For this review, take the finished solid that the model builds, in its own axes (mm). Face numbers are marked on the shaded views. A direction names the side the tool comes from. Coordinates: 2 decimals unless noted, no trailing zeros. Loops run counter-clockwise (first coordinate to the right, second up) from the corner with the lowest first, then second, coordinate; pieces in that order, holes last. Notation, with made-up numbers: (77, -28) -> (93, -28) arc R21 cw to (93, 6) -> close; hole circle Ø4 at (27.5, 65). An arc over 180 degrees is marked (long way). Answer in a Markdown table with one row per item.
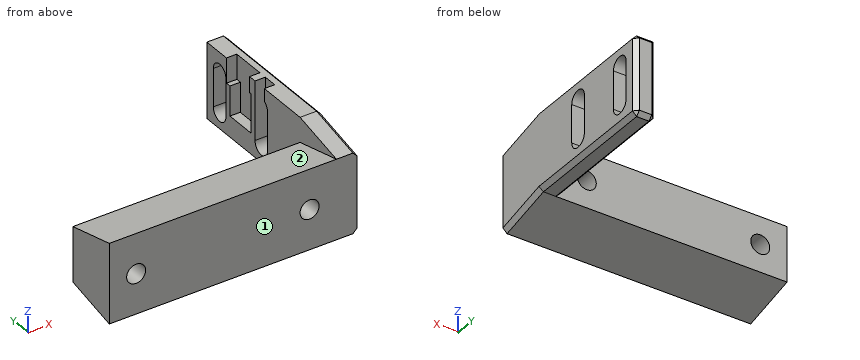
from build123d import *

# Parameters (mm, degrees)
PAD_DEPTH            = 55
SKETCH001_R          = 2.3
POCKET_DEPTH         = 13.001
PAD013_DEPTH         = 5
SKETCH023_W          = 7.25
SKETCH023_H          = 3.35
POCKET009_DEPTH      = 2.5
CHAMFER005_SIZE      = 1
BODY_PITCH_ANGLE     = 90
BODY_PLACEMENT_ANGLE = 90


with BuildPart() as part:
    # Sketch → Pad (new body)
    with BuildSketch(Plane.XZ):
        Polygon((0, 0), (19.3, 0), (16.3, 13), (3, 13), align=None)
    extrude(amount=PAD_DEPTH)

    # Sketch001 (on Face3 of Pad) → Pocket (cut, through all)
    with BuildSketch(Plane(origin=(0, 0, 13), x_dir=(-1, 0, 0), z_dir=(0, 0, 1))):
        with Locations((-9.65, 6.5)):
            Circle(SKETCH001_R)
        with Locations((-9.65, 48.5)):
            Circle(SKETCH001_R)
    extrude(amount=-POCKET_DEPTH, mode=Mode.SUBTRACT)

    # Sketch022 (on Face4 of Pocket) → Pad013 (join)
    with BuildSketch(Plane.XZ.offset(55)):
        Polygon((16.3, 13), (19.3, 0), (0, 0), (-3, 13), (-3, 47.3), (16.3, 47.3), (16.3, 44.3), (16.3, 24.3), (16.3, 18.3), align=None)
        with BuildLine():
            ThreePointArc((2.05, 44), (-0.2, 41.75), (2.05, 39.5))
            Line((2.05, 39.5), (11.25, 39.5))
            ThreePointArc((11.25, 39.5), (13.5, 41.75), (11.25, 44))
            Line((2.05, 44), (11.25, 44))
        make_face(mode=Mode.SUBTRACT)
        with BuildLine():
            ThreePointArc((2.05, 29.1), (-0.2, 26.85), (2.05, 24.6))
            Line((2.05, 24.6), (11.25, 24.6))
            ThreePointArc((11.25, 24.6), (13.5, 26.85), (11.25, 29.1))
            Line((2.05, 29.1), (11.25, 29.1))
        make_face(mode=Mode.SUBTRACT)
    extrude(amount=PAD013_DEPTH)

    # Sketch023 (on Face6 of Pad013) → Pocket009 (cut)
    with BuildSketch(Plane(origin=(0, -55, 0), x_dir=(1, 0, 0), z_dir=(0, 1, 0))):
        Polygon((10.25, -30.55), (10.25, -38.05), (3.05, -38.05), (3.05, -39.3), (-3, -39.3), (-3, -31.05), (0.85, -31.05), (0.85, -30.55), align=None)
        with Locations((0.625, -27.425)):
            Rectangle(SKETCH023_W, SKETCH023_H)
    extrude(amount=-POCKET009_DEPTH, mode=Mode.SUBTRACT)

    # Chamfer005
    chamfer005_edges = [part.edges().sort_by_distance(p)[0] for p in [
        (16.3, -57.5, 47.3),
        (6.65, -60, 47.3),
        (6.65, -55, 47.3),
        (-3, -57.5, 47.3),
        (-3, -60, 30.15),
        (16.3, -60, 30.15),
        (-1.5, -60, 6.5),
        (17.8, -60, 6.5),
        (16.3, -55, 30.15),
    ]]
    chamfer(chamfer005_edges, length=CHAMFER005_SIZE)


with BuildPart() as part_1:
    # Body pitch: moved
    add(part.part.rotate(Axis((0, 0, 0), (0, 1, 0)), BODY_PITCH_ANGLE))


with BuildPart() as part_2:
    # Body placement: moved
    add(part_1.part.moved(Location((-26, -25, -23))).rotate(Axis((-26, -25, -23), (0, 0, 1)), BODY_PLACEMENT_ANGLE))


solid = part_2.part
Item 1: For the marked faces 1 and 2, list the 3-axis set-ups (+Z, -Z, +X, -X, +Y, -Y) from which the entire face can be reached by the end or side of a thin tool; tool diameter is ignored.
Worked answers:
| item | result |
|---|---|
| face 1 | +Z, -Z, +X, -X, -Y |
| face 2 | +Z, -X, +Y |
Item 2: Take a section at B-B, the plane z = -32.5. State the section outline as (x, y) points, and give its area (3 significant figures).
Worked answers:
| item | result |
|---|---|
| outline | (-26, -25) -> (-21.8, -25) -> (-21.8, -12) -> (-26, -12) -> close; (-17.2, -25) -> (20.2, -25) -> (20.2, -12) -> (-17.2, -12) -> close; (24.8, -25) -> (34, -25) -> (34, -0.4) -> (29, -0.4) -> (29, -12) -> (24.8, -12) -> close; (29, 4.1) -> (34, 4.1) -> (34, 14.5) -> (29, 14.5) -> (29, 13.05) -> (31.5, 13.05) -> (31.5, 5.55) -> (29, 5.55) -> close; (29, 19) -> (34, 19) -> (34, 21.3) -> (33, 22.3) -> (30, 22.3) -> (29, 21.3) -> close |
| area | 767 mm² |
Item 3: Insertion check: pin 1 (1.3 mm diameter, centred on x = 30, y = 10, fed in from +Z); pin 2 (1.5 mm diameter, centred on x = 31, y = 7.5, fed in from -Z); pin 3 (2.5 mm diameter, centred on y = 3, z = -23, fed in from -X). Each pin has a flat end and moves straight along its axis. Give the tip position at first contact, or say it passes through.
Worked answers:
| item | result |
|---|---|
| pin 1 | z = -33.25 |
| pin 2 | z = -39.3 |
| pin 3 | x = 29 |
Item 4: Take a section at A-A, the plane y = 1.85. State the section outline as (x, z) points, and give its area (3 significant figures).
Worked answers:
| item | result |
|---|---|
| outline | (29, -38.3) -> (30, -39.3) -> (33, -39.3) -> (34, -38.3) -> (34, -36.5) -> (29, -36.5) -> close; (31.5, -22.8) -> (34, -22.8) -> (34, -21) -> (33, -20) -> (31.5, -20) -> close |
| area | 19.5 mm² |
Item 5: For L1, parallel to X at y = -19, z = -32.65; L2, parallel to X at y = 7.5, z = -33; L3, parallel to Y at x = 18.5, z = -27.25, list the stretches that pass through material, from the lowest coordinate up.
Worked answers:
| item | result |
|---|---|
| L1 | -26 to -21.8, -17.2 to 20.2, 24.8 to 34 |
| L2 | 31.5 to 34 |
| L3 | -25 to -12 |
Item 6: Take a section at D-D, the plane x = 24. State the section outline as (y, z) points.
Worked answers:
| item | result |
|---|---|
| outline | (-25, -42.3) -> (-12, -39.3) -> (-12, -34.39) -> (-25, -34.39) -> close; (-25, -30.91) -> (-12, -30.91) -> (-12, -26) -> (-25, -23) -> close |
Item 7: Take a section at C-C, the plane y = 9.5. State the section outline as (x, z) points, and give its area (3 significant figures).
Worked answers:
| item | result |
|---|---|
| outline | (29, -38.3) -> (30, -39.3) -> (33, -39.3) -> (34, -38.3) -> (34, -21) -> (33, -20) -> (31.5, -20) -> (31.5, -33.25) -> (29, -33.25) -> close |
| area | 61.9 mm² |
